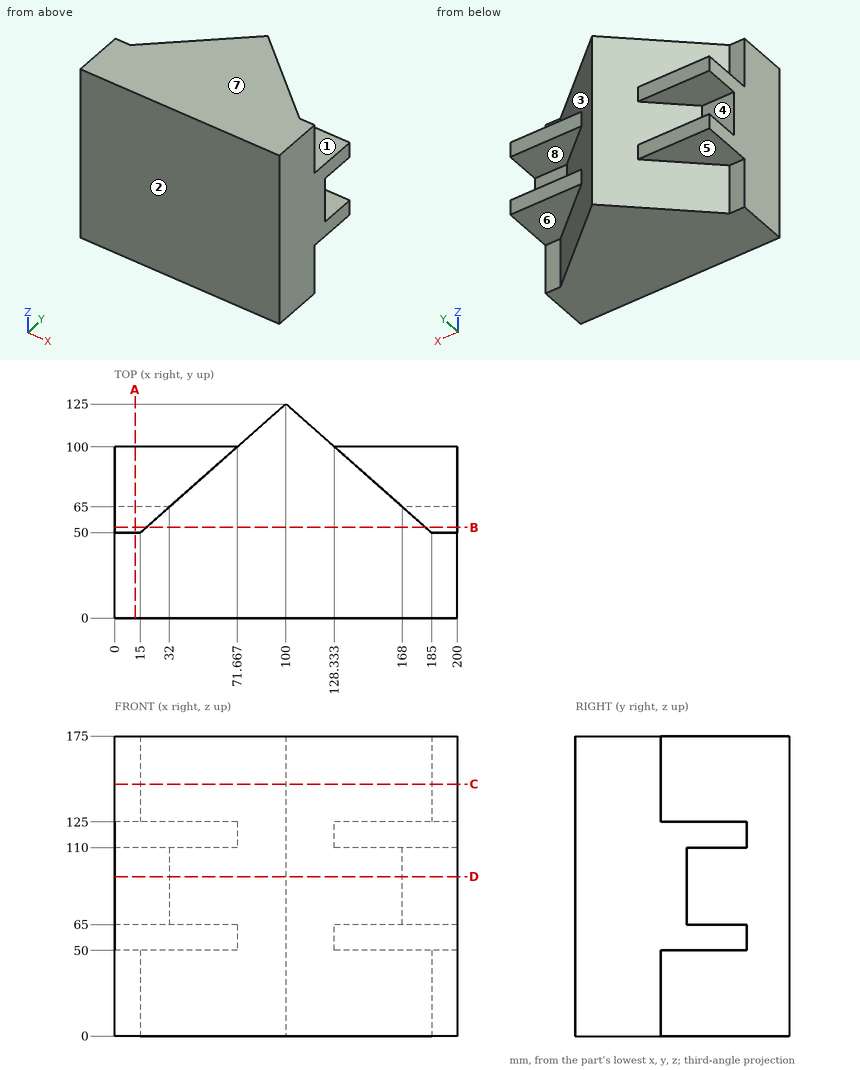
For this review, use the dimensioned drawing (mm, ordinates from the lowest corner) and the shaded views. A direction names the side the tool comes from. Round coordinates to 2 decimals unless told otherwise and drop trailing zeros. Loops run counter-clockwise (first coordinate to the right, second up) from the corner with the lowest first, then second, coordinate; pieces in that order, holes last. Notation, with made-up numbers: (-5.5, -32.5) -> (45.5, -32.5) arc R17 ccw to (45.5, 0.5) -> close; hole circle Ø5 at (0.5, -21). An arc over 180 degrees is marked (long way). Write item = value, one per line. Start each with the question number.
Item 1: Insertion check: pin 1 (4.5 mm diameter, centred on x = 174.5, z = 120.5, fed in from +Y); pin 2 (2 mm diameter, centred on x = 20, y = 56, fed in from +Z); pin 3 (12 mm diameter, centred on x = 189, z = 138.5, fed in from +Y) (1 decimal). Each pin has a flat end and moves straight along its axis. Give the tip position at first contact, or say it passes through.
Item 2: Take a section at A-A on x = 12. Give the boundary of the cut face in (y, z), plus the area to 3 significant figures.
Item 3: To check wall thickness, follow L1, parallel to Z at x = 26.5, y = 82.5; L2, parallel to Y at x = 190.5, z = 13; L3, parallel to Z at x = 185, y = 64.5. State the ranges of each line that lie inside material, in increasing order.
Item 4: Take a section at C-C on z = 147. Give the boundary of the cut face in (x, y), plus the area to 3 significant figures.
Item 5: Mouldability with a two-part tool opening along Z and no side actions: class the marked faces 1, 2 and 3 as released by +Z, released by -Z, zero draft, split by the parting line, or undercut.
Item 6: Take a section at B-B on y = 53. Give the boundary of the cut face in (x, z).
Item 7: For the marked faces 4, 5, 6, 7 and 8, list the 3-axis set-ups (+Z, -Z, +X, -X, +Y, -Y) from which the entire face can be reached by the end or side of a thin tool; tool diameter is ignored.
Item 8: Take a section at D-D on z = 93. Give the boundary of the cut face in (x, y), plus the area to 3 significant figures.
Result:
q1.pin_1 = 100
q1.pin_2 = 125
q1.pin_3 = 51.8
q2.outline = (0, 0) -> (50, 0) -> (50, 50) -> (100, 50) -> (100, 65) -> (65, 65) -> (65, 110) -> (100, 110) -> (100, 125) -> (50, 125) -> (50, 175) -> (0, 175) -> close
q2.area = 10,900 mm²
q3.L1 = 50 to 65, 110 to 125
q3.L2 = 0 to 50
q3.L3 = 50 to 125
q4.outline = (0, 0) -> (200, 0) -> (200, 50) -> (185, 50) -> (100, 125) -> (15, 50) -> (0, 50) -> close
q4.area = 16,400 mm²
q5.face_1 = released by +Z
q5.face_2 = zero draft
q5.face_3 = undercut
q6.outline = (0, 50) -> (18.4, 50) -> (18.4, 0) -> (181.6, 0) -> (181.6, 50) -> (200, 50) -> (200, 125) -> (181.6, 125) -> (181.6, 175) -> (18.4, 175) -> (18.4, 125) -> (0, 125) -> close
q7.face_4 = -X, +Y
q7.face_5 = -Z, -X, +Y
q7.face_6 = -Z, +X, +Y
q7.face_7 = +Z, +X, -X, +Y, -Y
q7.face_8 = +X, +Y
q8.outline = (0, 0) -> (200, 0) -> (200, 65) -> (168, 65) -> (100, 125) -> (32, 65) -> (0, 65) -> close
q8.area = 17,100 mm²
